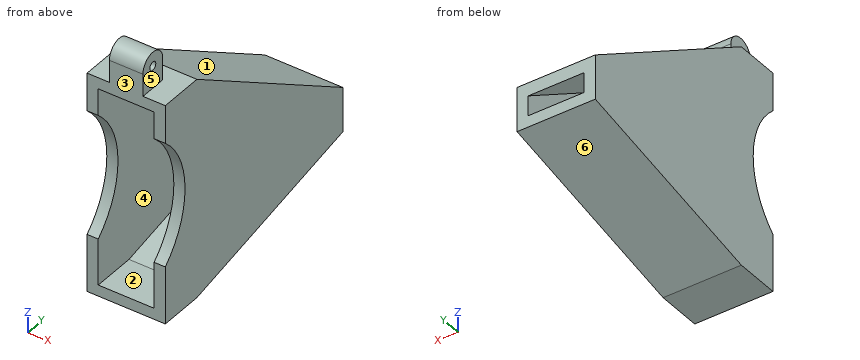
```python
from build123d import *

# Parameters (mm, degrees)
F1_DEPTH = 7
F2_T     = -2
F3_R     = 0.75
F4_DEPTH = 3


# Not quite as in the source:
# - a feature names something its author has since deleted; it is built from what else it names


with BuildPart() as f1:
    # F0 (on Right) → F1 (new body, symmetric)
    with BuildSketch(Plane.YZ):
        with BuildLine():
            Line((45, 8), (45, 16))
            Line((45, 16), (8, 39.5))
            Line((8, 39.5), (0, 39.5))
            Line((0, 39.5), (0, 32.6803398875))
            ThreePointArc((0, 32.6803398875), (5, 21.5), (0, 10.3196601125))
            Line((0, 10.3196601125), (0, 0))
            Line((0, 0), (8, 0))
            Line((8, 0), (45, 8))
        make_face()
    extrude(amount=F1_DEPTH, both=True)

    # F2
    f2_openings = [f1.faces().sort_by_distance(p)[0] for p in [
        (0, 0, 36.09017),
        (0, 5, 21.5),
        (0, 0, 5.15983),
        (0, 45, 12),
    ]]
    offset(amount=F2_T, openings=f2_openings)

    # F3 (on Right) → F4 (join, symmetric)
    with BuildSketch(Plane.YZ):
        with BuildLine():
            Line((0, 39.5), (5, 39.5))
            Line((5, 39.5), (5, 43.5))
            ThreePointArc((5, 43.5), (2.5, 46), (0, 43.5))
            Line((0, 43.5), (0, 39.5))
        make_face()
        with Locations((2.5, 43.5)):
            Circle(F3_R, mode=Mode.SUBTRACT)
    extrude(amount=F4_DEPTH, both=True)


solid = f1.part
```
Read the model definition and answer for the solid it produces. Units are mm, in the model's axes. Face numbers are marked on the shaded views. A direction names the side the tool comes from. Give positions to 0.01 mm unless a question says otherwise; leave off trailing zeros. Loops run counter-clockwise (first coordinate to the right, second up) from the corner with the lowest first, then second, coordinate; pieces in that order, holes last.
Item 1: The part is cut by section C-C (y = 30.5). Write down the section's boundary in (x, z).
Item 2: The part is cut by section D-D (y = 42). Write down the section's boundary in (x, z), and give its area (3 significant figures).
Item 3: The part is cut by section B-B (y = 2.5). Write down the section's boundary in (x, z).
Item 4: For the marked faces 4, 5 and 6, determine the directions among +Z, -Z, +X, -X, +Y, -Y from which every point of the face is accessible in a straight line to the end or side of a thin tool.
Item 5: Find the intervals of material crossed by line 1 along Z through (x, y) = (1.25, 2.5); line 2 along X through (y, z) = (22, 27); line 3 along Z through (x, y) = (0, 4.5), in increasing order.
Item 6: The part is cut by section A-A (x = -4.25). Write down the section's boundary in (y, z), and give its area (3 significant figures).
Item 7: The mould has two halves that part along Z. Classify the marked faces 1, 2 and 3: released by +Z, released by -Z, zero draft, split by the parting line, or undercut.
Item 8: Each of these flat-tipped pins is pushed along its axis until it touches: pin 1 Ø3 at (x, y) = (3, 38) entering from -Z; pin 2 Ø8 at (x, y) = (-3, 19.5) entering from -Z; pin 3 Ø2.5 at (y, z) = (2, 43.5) entering from -X; pin 4 Ø2 at (y, z) = (37.5, 24) entering from -X. Where does it stop, or does it pass through?
Taken from the geometry:
1. outline: (-7, 4.86) - (7, 4.86) - (7, 25.21) - (-7, 25.21) - close; hole (-5, 6.91) - (5, 6.91) - (5, 22.84) - (-5, 22.84) - close
2. outline: (-7, 7.35) - (7, 7.35) - (7, 17.91) - (-7, 17.91) - close; hole (-5, 9.4) - (5, 9.4) - (5, 15.54) - (-5, 15.54) - close
2. area: 86.4 mm2
3. outline: (-7, 0) - (7, 0) - (7, 13.21) - (5, 13.21) - (5, 2) - (-5, 2) - (-5, 13.21) - (-7, 13.21) - close; (-7, 29.79) - (-5, 29.79) - (-5, 37.5) - (5, 37.5) - (5, 29.79) - (7, 29.79) - (7, 39.5) - (3, 39.5) - (3, 42.75) - (-3, 42.75) - (-3, 39.5) - (-7, 39.5) - close; (-3, 44.25) - (3, 44.25) - (3, 46) - (-3, 46) - close
4. face 4: -Y
4. face 5: +Z, +X, +Y, -Y
4. face 6: -Z, +X, -X, +Y
5. line 1: z = 0 to 2, 37.5 to 42.75, 44.25 to 46
5. line 2: x = -7 to -5, 5 to 7
5. line 3: z = 0 to 2, 37.5 to 45
6. outline: (0, 0) - (8, 0) - (45, 8) - (45, 10.05) - (7.79, 2) - (0, 2) - close; (0, 37.5) - (7.42, 37.5) - (45, 13.63) - (45, 16) - (8, 39.5) - (0, 39.5) - close
6. area: 195 mm2
7. face 1: released by +Z
7. face 2: undercut
7. face 3: zero draft
8. pin 1: stops at z = 6.16
8. pin 2: stops at z = 1.62
8. pin 3: stops at x = -3
8. pin 4: passes through
